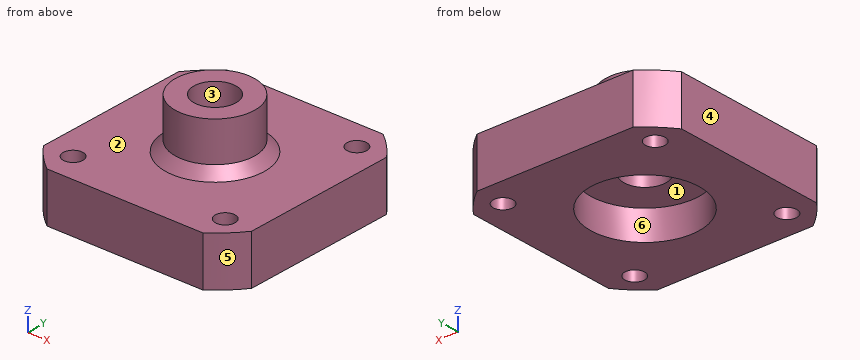
```python
from build123d import *

# Parameters (mm, degrees)
PAD_DEPTH       = 10
SKETCH_R        = 13
SKETCH_R_2      = 4.25
PAD001_DEPTH    = 20
PAD001_FACE22_R = 4.25
POCKET_DEPTH    = 6
SKETCH001_R     = 2
POCKET001_DEPTH = 10.0010008506
SKETCH002_R     = 16.036471
SKETCH002_R_2   = 8
POCKET002_DEPTH = 10
CHAMFER_SIZE    = 2


with BuildPart() as part:
    # Binder Face3 → Pad (new)
    with BuildSketch(Plane(origin=(80.0089996426, 399.2090804087, 169.428643648), x_dir=(0, 1, -2.4e-09), z_dir=(-1.8e-08, 2.4e-09, 1))):
        with BuildLine():
            Line((-21.2090002282, 15.8879926146), (-21.2089997718, -15.8879932238))
            ThreePointArc((-21.2089997718, -15.8879932238), (-18.7383294323, -18.7383299706), (-15.8879926146, -21.2090002282))
            Line((-15.8879926146, -21.2090002282), (15.8879932238, -21.2089997718))
            ThreePointArc((15.8879932238, -21.2089997718), (18.7383299706, -18.7383294323), (21.2090002282, -15.8879926146))
            Line((21.2090002282, -15.8879926146), (21.2089997718, 15.8879932238))
            ThreePointArc((21.2089997718, 15.8879932238), (18.7383294323, 18.7383299706), (15.8879926146, 21.2090002282))
            Line((15.8879926146, 21.2090002282), (-15.8879932238, 21.2089997718))
            ThreePointArc((-15.8879932238, 21.2089997718), (-18.7383299706, 18.7383294323), (-21.2090002282, 15.8879926146))
        make_face()
        with BuildLine():
            ThreePointArc((-15.4999997558, -17.0000002226), (-16.9999997774, -15.5000002442), (-15.4999997989, -14.0000002226))
            ThreePointArc((-15.4999997989, -14.0000002226), (-13.9999997774, -15.5000002011), (-15.4999997558, -17.0000002226))
        make_face(mode=Mode.SUBTRACT)
        with BuildLine():
            ThreePointArc((15.5000002442, -16.9999997774), (14.0000002226, -15.4999997989), (15.5000002011, -13.9999997774))
            ThreePointArc((15.5000002011, -13.9999997774), (17.0000002226, -15.4999997558), (15.5000002442, -16.9999997774))
        make_face(mode=Mode.SUBTRACT)
        with BuildLine():
            ThreePointArc((15.4999997989, 14.0000002226), (13.9999997774, 15.5000002011), (15.4999997558, 17.0000002226))
            ThreePointArc((15.4999997558, 17.0000002226), (16.9999997774, 15.5000002442), (15.4999997989, 14.0000002226))
        make_face(mode=Mode.SUBTRACT)
        with BuildLine():
            ThreePointArc((-15.5000002011, 13.9999997774), (-17.0000002226, 15.4999997558), (-15.5000002442, 16.9999997774))
            ThreePointArc((-15.5000002442, 16.9999997774), (-14.0000002226, 15.4999997989), (-15.5000002011, 13.9999997774))
        make_face(mode=Mode.SUBTRACT)
        with BuildLine():
            ThreePointArc((1.58e-07, -11), (-11, -1.58e-07), (-1.58e-07, 11))
            ThreePointArc((-1.58e-07, 11), (11, 1.58e-07), (1.58e-07, -11))
        make_face(mode=Mode.SUBTRACT)
    extrude(amount=-PAD_DEPTH)

    # Sketch (on Face20 of Pad) → Pad001 (join)
    with BuildSketch(Plane(origin=(-2.8643e-06, 3.803e-07, 159.4286431629), x_dir=(1, 0, 1.8e-08), z_dir=(1.8e-08, -2.4e-09, -1))):
        with Locations((80.0090026866, -399.2090800045)):
            Circle(SKETCH_R)
        with Locations((80.0090026866, -399.2090800045)):
            Circle(SKETCH_R_2, mode=Mode.SUBTRACT)
    extrude(amount=-PAD001_DEPTH)

    # Pad001 Face22 → Pocket (cut)
    with BuildSketch(Plane(origin=(80.0089998223, 399.2090803848, 159.428643648), x_dir=(0, -1, 2.4e-09), z_dir=(1.8e-08, -2.4e-09, -1))):
        with BuildLine():
            ThreePointArc((1.58e-07, 11), (-11, 1.58e-07), (-1.58e-07, -11))
            ThreePointArc((-1.58e-07, -11), (11, -1.58e-07), (1.58e-07, 11))
        make_face()
        Circle(PAD001_FACE22_R, mode=Mode.SUBTRACT)
    extrude(amount=-POCKET_DEPTH, mode=Mode.SUBTRACT)

    # Sketch001 (on Face3 of Pocket) → Pocket001 (cut, through all)
    with BuildSketch(Plane(origin=(-3.0439e-06, 4.042e-07, 169.4286431629), x_dir=(1, 0, 1.8e-08), z_dir=(-1.8e-08, 2.4e-09, 1))):
        with Locations((64.509002464, 414.7090797819)):
            Circle(SKETCH001_R)
        with Locations((95.509002464, 414.7090802271)):
            Circle(SKETCH001_R)
        with Locations((95.5090029092, 383.7090802271)):
            Circle(SKETCH001_R)
        with Locations((64.5090029092, 383.7090797819)):
            Circle(SKETCH001_R)
    extrude(amount=-POCKET001_DEPTH, mode=Mode.SUBTRACT)

    # Sketch002 (on Face16 of Pocket001) → Pocket002 (cut)
    with BuildSketch(Plane(origin=(-3.2236e-06, 4.28e-07, 179.4286431629), x_dir=(1, 0, 1.8e-08), z_dir=(-1.8e-08, 2.4e-09, 1))):
        with Locations((80.0090026866, 399.2090800045)):
            Circle(SKETCH002_R)
        with Locations((80.0090026866, 399.2090800045)):
            Circle(SKETCH002_R_2, mode=Mode.SUBTRACT)
    extrude(amount=-POCKET002_DEPTH, mode=Mode.SUBTRACT)

    # Chamfer
    chamfer_edges = [part.edges().sort_by_distance(p)[0] for p in [
        (72.009, 399.20908, 169.428644),
    ]]
    chamfer(chamfer_edges, length=CHAMFER_SIZE)


solid = part.part
```
Work out the finished part from the listing and answer in its coordinate system (mm). Face numbers are marked on the shaded views. A direction names the side the tool comes from. Coordinates: 2 decimals unless noted, no trailing zeros. Loops run counter-clockwise (first coordinate to the right, second up) from the corner with the lowest first, then second, coordinate; pieces in that order, holes last. Notation, with made-up numbers: (13.25, -24) - (62.25, -24) arc R28 cw to (62.25, 15) - close; hole circle Ø8 at (-5.75, 10). An arc over 180 degrees is marked (long way). Use a Markdown table: item, result.
Item 1: Given pin 1 Ø6 at (x, z) = (77, 174.5) entering from -Y; pin 2 Ø2 at (y, z) = (391.5, 172.5) entering from -X; pin 3 Ø10 at (x, z) = (90.5, 171) entering from -Y; pin 4 Ø11 at (x, y) = (82.5, 399.5) entering from -Z, each flat-ended and moving along its own axis, determine where each tip first touches the part or whether it passes through.
Evaluation:
| item | result |
|---|---|
| pin 1 | stops at y = 391.21 |
| pin 2 | stops at x = 75.65 |
| pin 3 | stops at y = 378 |
| pin 4 | stops at z = 165.43 |
Item 2: For the marked faces 1, 2 and 3, determine the directions among +Z, -Z, +X, -X, +Y, -Y from which every point of the face is accessible in a straight line to the end or side of a thin tool.
Evaluation:
| item | result |
|---|---|
| face 1 | -Z |
| face 2 | +Z |
| face 3 | +Z, -Z |
Item 3: Find section C-C, the plane y = 411. Determine the outline of the cut face in (x, z), and give its area (3 significant figures).
Evaluation:
| item | result |
|---|---|
| outline | (58.8, 159.43) - (101.22, 159.43) - (101.22, 169.43) - (58.8, 169.43) - close |
| area | 424 mm2 |
Item 4: Consider probe 1 along Z at (x, y) = (94, 398); probe 2 along Z at (x, y) = (90, 398); probe 3 along Y at (x, z) = (79, 172.5). Determine where each line is inside the solid, lowest interval first. Write a range as from..to.
Evaluation:
| item | result |
|---|---|
| probe 1 | z = 159.43..169.43 |
| probe 2 | z = 165.43..169.43 |
| probe 3 | y = 391.27..395.08, 403.34..407.15 |
Item 5: The mould has two halves that part along X. Classify the marked faces 4, 5 and 6: +X half, -X half, draft (parallel to the pull), parting line (faces both ways), or undercut.
Evaluation:
| item | result |
|---|---|
| face 4 | -X half |
| face 5 | +X half |
| face 6 | undercut |
Item 6: Find section A-A, the plane x = 65.5. Determine the outline of the cut face in (y, z).
Evaluation:
| item | result |
|---|---|
| outline | (378, 159.43) - (381.97, 159.43) - (381.97, 169.43) - (378, 169.43) - close; (385.45, 159.43) - (412.97, 159.43) - (412.97, 169.43) - (385.45, 169.43) - close; (416.45, 159.43) - (420.42, 159.43) - (420.42, 169.43) - (416.45, 169.43) - close |
Item 7: Find section B-B, the plane z = 178.25. Determine the outline of the cut face in (x, y).
Evaluation:
| item | result |
|---|---|
| outline | circle Ø16 at (80.01, 399.21); hole circle Ø8.5 at (80.01, 399.21) |
Item 8: Find section D-D, the plane z = 162.25. State how many separate pieces and enclosed holes the cut face has, and give its area (3 significant figures).
Evaluation:
| item | result |
|---|---|
| separate pieces | 1 |
| enclosed holes | 5 |
| area | 1,320 mm2 |
